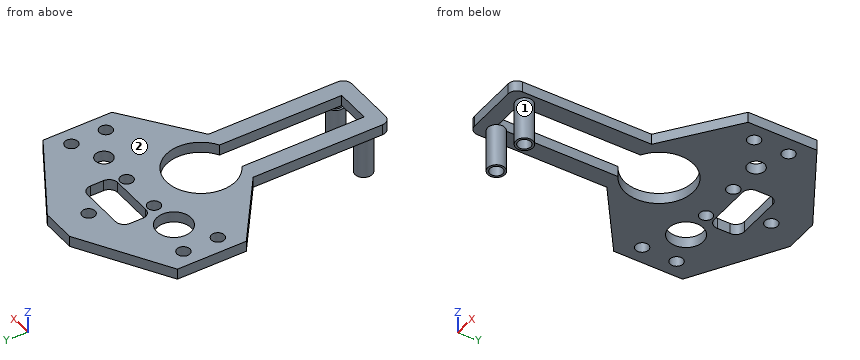
from build123d import *

# Parameters (mm, degrees)
SKETCH1_R           = 4
SKETCH1_R_2         = 1.5
SKETCH1_R_3         = 2
BOSS_EXTRUDE1_DEPTH = 2.5
SKETCH2_R           = 2
SKETCH2_R_2         = 1.5
BOSS_EXTRUDE2_DEPTH = 10
FILLET1_R           = 2


with BuildPart() as part:
    # Sketch1 → Boss-Extrude1 (new body)
    with BuildSketch(Plane.XY):
        Polygon((-24, 5.07179677), (-24, 21.07179677), (-4, 33.07179677), (4, 33.07179677), (24, 21.07179677), (24, 5.07179677), (8, -6.92820323), (8, -38.92820323), (-8, -38.92820323), (-8, -6.92820323), align=None)
        with Locations((-12, 14.07179677)):
            Circle(SKETCH1_R, mode=Mode.SUBTRACT)
        with Locations((-4.875, 14.07179677)):
            Circle(SKETCH1_R_2, mode=Mode.SUBTRACT)
        with Locations((4.875, 14.07179677)):
            Circle(SKETCH1_R_2, mode=Mode.SUBTRACT)
        with Locations((0, 26.07179677)):
            Circle(SKETCH1_R_2, mode=Mode.SUBTRACT)
        with Locations((20, 17.07179677)):
            Circle(SKETCH1_R_2, mode=Mode.SUBTRACT)
        with Locations((20, 9.07179677)):
            Circle(SKETCH1_R_2, mode=Mode.SUBTRACT)
        with Locations((-20, 17.07179677)):
            Circle(SKETCH1_R_2, mode=Mode.SUBTRACT)
        with Locations((-20, 9.07179677)):
            Circle(SKETCH1_R_2, mode=Mode.SUBTRACT)
        with Locations((13, 14.07179677)):
            Circle(SKETCH1_R_3, mode=Mode.SUBTRACT)
        with BuildLine():
            Line((-4, -35.29820323), (4, -35.29820323))
            Line((4, -35.29820323), (4, -6.92820323))
            ThreePointArc((4, -6.92820323), (0, 8), (-4, -6.92820323))
            Line((-4, -6.92820323), (-4, -35.29820323))
        make_face(mode=Mode.SUBTRACT)
        with BuildLine():
            Line((-5, 23.07179677), (5, 23.07179677))
            ThreePointArc((5, 23.07179677), (6.414213562, 22.486010332), (7, 21.07179677))
            Line((7, 21.07179677), (7, 18.07179677))
            ThreePointArc((7, 18.07179677), (6.414213562, 16.657583207), (5, 16.07179677))
            Line((5, 16.07179677), (-5, 16.07179677))
            ThreePointArc((-5, 16.07179677), (-6.414213562, 16.657583207), (-7, 18.07179677))
            Line((-7, 18.07179677), (-7, 21.07179677))
            ThreePointArc((-7, 21.07179677), (-6.414213562, 22.486010332), (-5, 23.07179677))
        make_face(mode=Mode.SUBTRACT)
    extrude(amount=BOSS_EXTRUDE1_DEPTH)

    # Sketch2 → Boss-Extrude2 (add)
    # profile 1 of 2: a face of its own
    with BuildSketch(Plane(origin=(0, 0, 0), x_dir=(-1, 0, 0), z_dir=(0, 0, -1))):
        with Locations(Location((-5, -34.53164975, 0), (0, 0, 60))):
            Circle(SKETCH2_R)
        with Locations(Location((-5, -34.53164975, 0), (0, 0, 48.189685104))):
            Circle(SKETCH2_R_2, mode=Mode.SUBTRACT)
    # profile 2 of 2: a face of its own
    with BuildSketch(Plane(origin=(0, 0, 0), x_dir=(-1, 0, 0), z_dir=(0, 0, -1))):
        with Locations(Location((5, -34.53164975, 0), (0, 0, 180))):
            Circle(SKETCH2_R)
        with Locations(Location((5, -34.53164975, 0), (0, 0, 180))):
            Circle(SKETCH2_R_2, mode=Mode.SUBTRACT)
    extrude(amount=BOSS_EXTRUDE2_DEPTH)

    # Fillet1
    fillet1_edges = [part.edges().sort_by_distance(p)[0] for p in [
        (8, -38.92820323, 1.25),
        (-8, -38.92820323, 1.25),
    ]]
    fillet(fillet1_edges, radius=FILLET1_R)


solid = part.part
Work out the finished part from the listing and answer in its coordinate system (mm). Face numbers are marked on the shaded views. Round coordinates to 2 decimals unless told otherwise and drop trailing zeros. Write each loop counter-clockwise with the first axis right and the second up, starting at its lowest first coordinate (ties: lowest second). Pieces come first, ordered by that corner, then holes.
1) A cutting plane is placed at C-C (x = -20). Give the vertices of the cut face in (y, z).
2) A cutting plane is placed at A-A (x = 0). Give the vertices of the cut face in (y, z), plus the area to 3 significant figures.
3) A cutting plane is placed at D-D (z = -6.25). Give the vertices of the cut face in (x, y).
4) Given pin 1 Ø4 at (x, y) = (-13.5, -4) entering from +Z; pin 2 Ø24 at (x, y) = (5.5, -1) entering from -Z; pin 3 Ø0.8 at (y, z) = (-17, 1) entering from -X; pin 4 Ø0.8 at (x, y) = (3.5, -34.5) entering from +Z, each flat-ended and moving along its own axis, determine where each tip first touches the part or whether it passes through.
5) A cutting plane is placed at B-B (y = 6.5). Give the vertices of the cut face in (x, z), plus the area to 3 significant figures.
6) Straight lines are drawn through the part: line 1 (Y direction, x = 0, z = 0.9); line 2 (X direction, y = -9.5, z = 1.5); line 3 (Y direction, x = 20, z = 1.4). For each, find the intervals that lie inside material, in ascending order.
7) The mould has two halves that part along X. Classify the marked faces 1 and 2: pulls with the +X half, pulls with the -X half, needs draft (parallel to the pull), parting line crosses it, or undercut.
Completed:
1. outline: (2.07, 0) - (7.57, 0) - (7.57, 2.5) - (2.07, 2.5) - close; (10.57, 0) - (15.57, 0) - (15.57, 2.5) - (10.57, 2.5) - close; (18.57, 0) - (23.47, 0) - (23.47, 2.5) - (18.57, 2.5) - close
2. outline: (-38.93, 0) - (-35.3, 0) - (-35.3, 2.5) - (-38.93, 2.5) - close; (8, 0) - (16.07, 0) - (16.07, 2.5) - (8, 2.5) - close; (23.07, 0) - (24.57, 0) - (24.57, 2.5) - (23.07, 2.5) - close; (27.57, 0) - (33.07, 0) - (33.07, 2.5) - (27.57, 2.5) - close
2. area: 46.8 mm2
3. outline: circle Ø4 at (-5, -34.53); circle Ø4 at (5, -34.53); hole circle Ø3 at (-5, -34.53); hole circle Ø3 at (5, -34.53)
4. pin 1: stops at z = 2.5
4. pin 2: stops at z = 0
4. pin 3: stops at x = -8
4. pin 4: stops at z = 0
5. outline: (-24, 0) - (-4.66, 0) - (-4.66, 2.5) - (-24, 2.5) - close; (4.66, 0) - (24, 0) - (24, 2.5) - (4.66, 2.5) - close
5. area: 96.7 mm2
6. line 1: y = -38.93 to -35.3, 8 to 16.07, 23.07 to 24.57, 27.57 to 33.07
6. line 2: x = -8 to -4, 4 to 8
6. line 3: y = 2.07 to 7.57, 10.57 to 15.57, 18.57 to 23.47
7. face 1: undercut
7. face 2: needs draft
